from build123d import *

# Parameters (mm, degrees)
F0_W      = 52
F0_H      = 64
F1_DEPTH  = 50
F2_W      = 40
F2_H      = 40
F3_DEPTH  = 50
F4_W      = 26
F4_H      = 26
F5_DEPTH  = 5
F6_R      = 7
F7_DEPTH  = 40
F8_W      = 26
F8_H      = 26
F9_DEPTH  = 5
F10_R     = 7
F11_DEPTH = 25


with BuildPart() as f1:
    # F0 (on Top) → F1 (new body)
    with BuildSketch(Plane.XY):
        with Locations((26, 32)):
            Rectangle(F0_W, F0_H)
    extrude(amount=F1_DEPTH)

    # F2 (on face) → F3 (cut)
    with BuildSketch(Plane.XY.offset(50)):
        with Locations((26, 32)):
            Rectangle(F2_W, F2_H)
    extrude(amount=-F3_DEPTH, mode=Mode.SUBTRACT)

    # F4 (on face) → F5 (cut)
    with BuildSketch(Plane.XZ):
        with Locations((26, 25)):
            Rectangle(F4_W, F4_H)
    extrude(amount=-F5_DEPTH, mode=Mode.SUBTRACT)

    # F6 (on face) → F7 (cut)
    with BuildSketch(Plane.XZ.offset(-5)):
        with Locations((26, 25)):
            Circle(F6_R)
    extrude(amount=-F7_DEPTH, mode=Mode.SUBTRACT)

    # F8 (on face) → F9 (cut)
    with BuildSketch(Plane(origin=(0, 64, 0), x_dir=(-1, 0, 0), z_dir=(0, 1, 0))):
        with Locations((-26, 25)):
            Rectangle(F8_W, F8_H)
    extrude(amount=-F9_DEPTH, mode=Mode.SUBTRACT)

    # F10 (on face) → F11 (cut)
    with BuildSketch(Plane(origin=(0, 59, 0), x_dir=(-1, 0, 0), z_dir=(0, 1, 0))):
        with Locations((-26, 25)):
            Circle(F10_R)
    extrude(amount=-F11_DEPTH, mode=Mode.SUBTRACT)


solid = f1.part
Model file for the job. Use its own axes, mm. A direction names the side the tool comes from. Round coordinates to 2 decimals unless told otherwise and drop trailing zeros. Order: outer loops, then holes, each group sorted by start corner. A loop starts at its lowest first (then second) coordinate and runs counter-clockwise, first axis right, second up.
(1) Pull direction Z, two halves, no side cores. Call faces 1 (the face through (26, 11, 0)), 2 (the face through (26, 2, 38)), 3 (the face through (52, 32, 25)): released by +Z, released by -Z, zero draft, split by the parting line, or undercut.
(2) Band-saw the part on C-C (z = 25). List the corners of the cut face in (x, y).
(3) Band-saw the part on A-A (y = 34). List the corners of the cut face in (x, z).
(4) Band-saw the part on B-B (x = 26). List the corners of the cut face in (y, z).
(5) Pin check, flat tips, straight feed: pin 1 (12 mm diameter, centred on y = 18, z = 20, fed in from -X); pin 2 (22.5 mm diameter, centred on x = 26, z = 25, fed in from -Y); pin 3 (5 mm diameter, centred on x = 10, y = 28.5, fed in from -Z); pin 4 (16 mm diameter, centred on x = 26, z = 25, fed in from +Y). Stop position of each tip, or through.
(6) Band-saw the part on D-D (x = 7). List the corners of the cut face in (y, z), then the cut area to 3 significant figures.
(7) Drill centre lines: line 1 (Z direction, x = 22, y = 60); line 2 (X direction, y = 49, z = 34.5); line 3 (Z direction, x = 26, y = 54.25). Where is each one in solid material? Low to high.
(8) 3-axis set-ups, long thin cutter, end or side, ignore diameter. For faces 4 (the face through (13, 2, 25)), 5 (the face through (0, 32, 25)), 6 (the face through (39, 62, 25)), 7 (the face through (21, 52, 31)): which of +Z, -Z, +X, -X, +Y, -Y reach the whole face in a straight line?
Verdict:
1. face 1: released by -Z
1. face 2: undercut
1. face 3: zero draft
2. outline: (0, 0) - (13, 0) - (13, 5) - (19, 5) - (19, 12) - (6, 12) - (6, 52) - (19, 52) - (19, 59) - (13, 59) - (13, 64) - (0, 64) - close; (33, 5) - (39, 5) - (39, 0) - (52, 0) - (52, 64) - (39, 64) - (39, 59) - (33, 59) - (33, 52) - (46, 52) - (46, 12) - (33, 12) - close
3. outline: (0, 0) - (6, 0) - (6, 50) - (0, 50) - close; (46, 0) - (52, 0) - (52, 50) - (46, 50) - close
4. outline: (0, 0) - (12, 0) - (12, 18) - (5, 18) - (5, 12) - (0, 12) - close; (0, 38) - (5, 38) - (5, 32) - (12, 32) - (12, 50) - (0, 50) - close; (52, 0) - (64, 0) - (64, 12) - (59, 12) - (59, 18) - (52, 18) - close; (52, 32) - (59, 32) - (59, 38) - (64, 38) - (64, 50) - (52, 50) - close
5. pin 1: stops at x = 0
5. pin 2: stops at y = 5
5. pin 3: passes through
5. pin 4: stops at y = 59
6. outline: (0, 0) - (12, 0) - (12, 50) - (0, 50) - close; (52, 0) - (64, 0) - (64, 50) - (52, 50) - close
6. area: 1,200 mm2
7. line 1: z = 0 to 12, 38 to 50
7. line 2: x = 0 to 6, 46 to 52
7. line 3: z = 0 to 18, 32 to 50
8. face 4: -Y
8. face 5: +Z, -Z, -X, +Y, -Y
8. face 6: +Y
8. face 7: +Z, -Z
